Geometry: final body of the model. Coordinates: model frame, mm. Round coordinates to 2 decimals unless told otherwise and drop trailing zeros. Order: outer loops, then holes, each group sorted by start corner. A loop starts at its lowest first (then second) coordinate and runs counter-clockwise, first axis right, second up. Notation, with made-up numbers: (29, 69.5) - (58, 69.5) arc R19 cw to (58, 104.5) - close; hole circle Ø7 at (13.5, 68.5). An arc over 180 degrees is marked (long way). Put each result on its own line as item: value. Start each with the question number.
(1) Section D-D (y = -29). Output: boundary loops of the cut face in (x, z).
(2) Section C-C (x = 55.5). Output: boundary loops of the cut face in (y, z).
(3) Material intervals for L1, parallel to Y at x = 0, z = 7; L2, parallel to X at y = -47, z = 2.75; L3, parallel to X at y = 92, z = 1, sorted ascending. Write a range as [from, to].
(4) Pin query (flat end, axial travel): P1, Ø6, axis at y = 32, z = 6, coming from the +X side; P2, Ø3, axis at x = -79.5, z = 3, coming from the +Y side; P3, Ø14, axis at x = -80.11, y = -46.25, coming from the -Z side; P4, Ø7, axis at x = 80.11, y = -46.25, coming from the -Z side. Return the tip coordinate at first contact, or that it passes through.
(5) Pull-direction query (Y, two-part tool) for faces 1 (the face through (-112.39, -4.95, 4.93)), 2 (the face through (-2, 2, 0)), 3 (the face through (78.81, 52.11, 4.93)); classes: released by +Y, released by -Y, zero draft, split by the parting line, or undercut.
(6) Section B-B (y = 46.25). Output: boundary loops of the cut face in (x, z).
(7) Section A-A (z = 6.75). Output: boundary loops of the cut face in (x, y), and give its area (3 significant figures).
Autodesk Inventor part; units mm, degrees
ref_plane "YZ Plane" through (0, 0, 0) normal (1, 0, 0) x (0, 1, 0)
ref_plane "XZ Plane" through (0, 0, 0) normal (0, 1, 0) x (-1, 0, 0)
ref_plane "XY Plane" through (0, 0, 0) normal (0, 0, 1) x (1, 0, 0)
sketch "Sketch6" plane through (0, 0, 0) normal (0, 0, 1) x (1, 0, 0)
  circle A0 centre (0, 0) radius 72.5
  circle A1 centre (0, 0) radius 112.5
  dimension "d46" = 145
  dimension "d47" = 225
extrude "Plate1" add sketch "Sketch6" along normal blind 10 contours A0 | A1
sketch "Sketch8" plane through (0, 0, 0) normal (0, 0, -1) x (-1, 0, 0)
  circle A0 centre (0, 92.5) radius 6
  circle A1 centre (0, 0) radius 92.5 construction
  dimension "d51" = 185
  dimension "d50" = 12
extrude "Extrusion6" cut sketch "Sketch8" along normal through all both and the other way through all
pattern_circular "Circular Pattern3" count 6 over 360 about axis through (0, 0, 0) along (0, 0, 1) of "Extrusion6"
equation "\"d47\" = back_steel_circle_диам_центров + back_steel_circle_ширина_кольца"
equation "\"d51\" = back_steel_circle_диам_центров"
equation "\"d45\" = Thickness"
equation "\"BendReliefDepth\" = 0.5 * Thickness"
properties part number "NVPH-306 revision cup"
Checks:
1. outline: (-108.7, 0) - (108.7, 0) - (108.7, 10) - (-108.7, 10) - close
2. outline: (-97.86, 0) - (97.86, 0) - (97.86, 10) - (-97.86, 10) - close
3. L1: y = [-112.5, -98.5], [-86.5, 86.5], [98.5, 112.5]
3. L2: x = [-102.21, -86.06], [-74.15, 74.15], [86.06, 102.21]
3. L3: x = [-64.75, -5.98], [5.98, 64.75]
4. P1: stops at x = 108.7
4. P2: stops at y = 81.07
4. P3: stops at z = 0
4. P4: passes through
5. face 1: split by the parting line
5. face 2: zero draft
5. face 3: undercut
6. outline: (-102.55, 0) - (-86.11, 0) - (-86.11, 10) - (-102.55, 10) - close; (-74.11, 0) - (74.11, 0) - (74.11, 10) - (-74.11, 10) - close; (86.11, 0) - (102.55, 0) - (102.55, 10) - (86.11, 10) - close
7. outline: circle Ø225 at (0, 0); hole circle Ø12 at (-80.11, -46.25); hole circle Ø12 at (-80.11, 46.25); hole circle Ø12 at (0, -92.5); hole circle Ø12 at (0, 92.5); hole circle Ø12 at (80.11, -46.25); hole circle Ø12 at (80.11, 46.25)
7. area: 39,100 mm²
